Verification items for this drawing (mm, ordinates from the low corner). A direction names the side the tool comes from. Give positions to 0.01 mm unless a question says otherwise; leave off trailing zeros. Loops run counter-clockwise (first coordinate to the right, second up) from the corner with the lowest first, then second, coordinate; pieces in that order, holes last. Notation, with made-up numbers: M -17.75,36.5 L 4.25,36.5 A11 ccw 4.25,40.5 Z; hole C 26.25,11.25 d6. An arc over 180 degrees is marked long. Put each result on its own line as item: value. Start each with the question number.
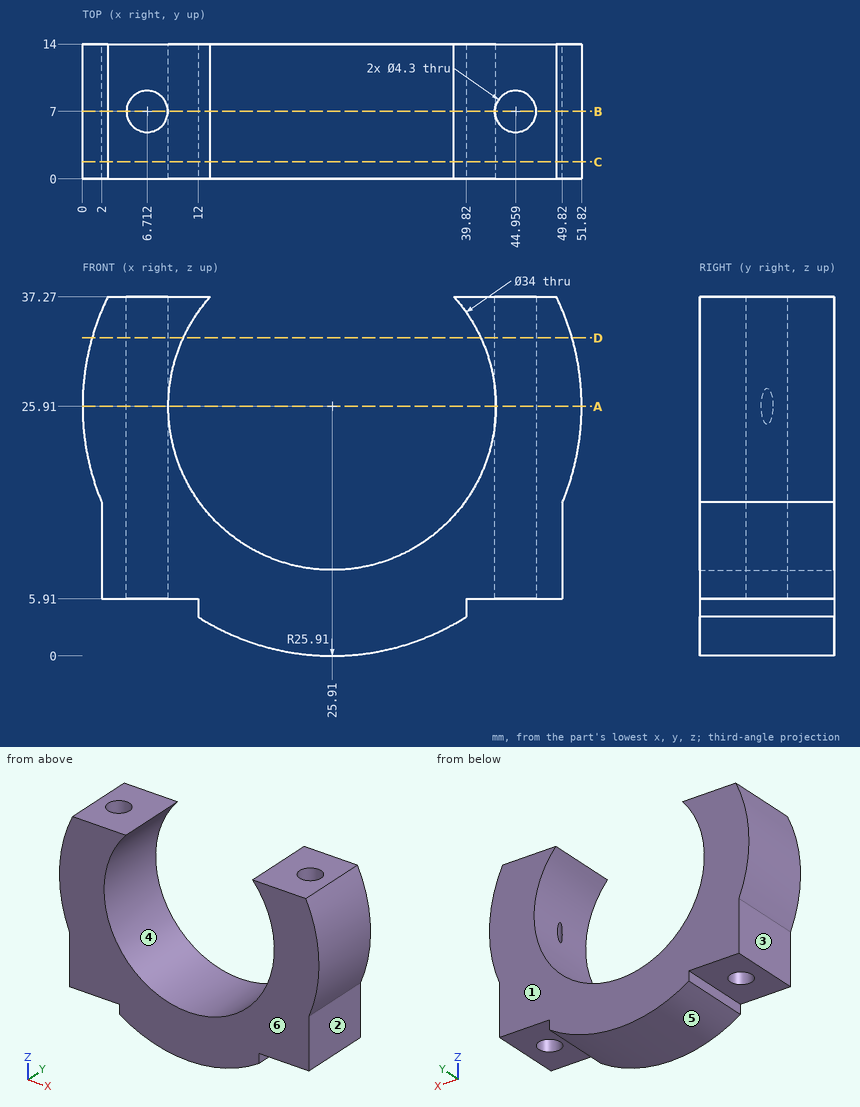
Q1. Scan lines: L1, parallel to Y at x = 45, z = 20.5; L2, parallel to X at y = 6, z = 22.5 (1 decimal); L3, parallel to X at y = 4, z = 25.5 (1 decimal). Record each from-to range of solid material in increasing order.
Q2. Set-up check for the marked faces 1, 2 and 3: record each of +Z, -Z, +X, -X, +Y, -Y from which the full face is reachable in a straight line by a thin tool's end or side.
Q3. Cross-section at B-B, the plane y = 7. Record the boundary of the cut face in (x, z), then the cut area to 3 significant figures.
Q4. Go/stop test with flat-tipped pins: pin 1 (5 mm diameter, centred on x = 21.5, y = 2.5, fed in from -Z); pin 2 (5 mm diameter, centred on y = 7.5, z = 10, fed in from +X); pin 3 (3 mm diameter, centred on y = 8.5, z = 12, fed in from -X). Record where each tip stops, or that it passes through.
Q5. Cross-section at C-C, the plane y = 1.75. Record the boundary of the cut face in (x, z).
Q6. Cross-section at D-D, the plane z = 33. Record the boundary of the cut face in (x, y).
Q7. Cross-section at A-A, the plane z = 25.91. Record the boundary of the cut face in (x, y).
Q8. Release check for a two-part mould opening along Z. For the marked faces 4, 5 and 6 record: pulls with the +Z half, pulls with the -Z half, needs draft (parallel to the pull), parting line crosses it, or undercut.
Ans:
1. L1: y = 0 to 4.85, 9.15 to 14
1. L2: x = 0.2 to 4.8, 8.6 to 9.3, 42.6 to 43.1, 46.9 to 51.6
1. L3: x = 0 to 8.9, 42.9 to 51.8
2. face 1: +Z, -Z, +X, -X, +Y
2. face 2: -Z, +X, +Y, -Y
2. face 3: -Z, -X, +Y, -Y
3. outline: M 2,5.91 L 4.56,5.91 L 4.56,37.27 L 2.62,37.27 A25.91 ccw 2,15.93 Z; M 8.86,5.91 L 12,5.91 L 12,4.05 A25.91 ccw 39.82,4.05 L 39.82,5.91 L 42.81,5.91 L 42.81,24.06 A17 cw long 13.26,37.27 L 8.86,37.27 Z; M 38.56,37.27 A17 cw 42.81,27.76 L 42.81,37.27 Z; M 47.11,5.91 L 49.82,5.91 L 49.82,15.93 A25.91 ccw 49.2,37.27 L 47.11,37.27 Z
3. area: 602 mm^2
4. pin 1: stops at z = 0.07
4. pin 2: stops at x = 49.82
4. pin 3: stops at x = 2
5. outline: M 2,5.91 L 12,5.91 L 12,4.05 A25.91 ccw 39.82,4.05 L 39.82,5.91 L 49.82,5.91 L 49.82,15.93 A25.91 ccw 49.2,37.27 L 38.56,37.27 A17 cw long 13.26,37.27 L 2.62,37.27 A25.91 ccw 2,15.93 Z
6. outline: M 0.99,0 L 10.46,0 L 10.46,14 L 0.99,14 Z; M 41.36,0 L 50.83,0 L 50.83,14 L 41.36,14 Z; hole C 6.71,7 d4.3; hole C 44.96,7 d4.3
7. outline: M 0,0 L 8.91,0 L 8.91,14 L 0,14 Z; M 42.91,0 L 51.82,0 L 51.82,14 L 42.91,14 L 42.91,7.65 A2.15 cw long 42.91,6.35 Z; hole C 6.71,7 d4.3
8. face 4: undercut
8. face 5: pulls with the -Z half
8. face 6: needs draft
